```python
from build123d import *

# Parameters (mm, degrees)
ESQUISSE1_W                  = 40
ESQUISSE1_H                  = 50
BOSS_EXTRU_1_DEPTH           = 10
ENL_V_MAT_EXTRU_1_DEPTH      = 65.807406984
ENL_V_MAT_EXTRU_1_DEPTH_BACK = 65.807406984
ESQUISSE2_R                  = 3.4
ESQUISSE2_R_2                = 3.5
CONG_1_R                     = 5


with BuildPart() as part:
    # Esquisse1 → Boss.-Extru.1 (new body)
    with BuildSketch(Plane.XY):
        with Locations((20, 25)):
            Rectangle(ESQUISSE1_W, ESQUISSE1_H)
    extrude(amount=BOSS_EXTRU_1_DEPTH)

    # Esquisse2 → Enlèv. mat.-Extru.1 (cut, two sides: drawn at the far end of the back side and taken through both)
    with BuildSketch(Plane.XY.offset(10).offset(-ENL_V_MAT_EXTRU_1_DEPTH_BACK)):
        with Locations((20, 25)):
            Circle(ESQUISSE2_R)
        with Locations((20, 7.5)):
            Circle(ESQUISSE2_R_2)
        with Locations(Location((20, 42.5, 0), (0, 0, 180))):
            Circle(ESQUISSE2_R_2)
    extrude(amount=ENL_V_MAT_EXTRU_1_DEPTH + ENL_V_MAT_EXTRU_1_DEPTH_BACK, mode=Mode.SUBTRACT)

    # Congé1
    cong_1_edges = [part.edges().sort_by_distance(p)[0] for p in [
        (0, 50, 5),
        (40, 50, 5),
        (40, 0, 5),
        (0, 0, 5),
    ]]
    fillet(cong_1_edges, radius=CONG_1_R)


solid = part.part
```
Work out the finished part from the listing and answer in its coordinate system (mm). Give positions to 0.01 mm unless a question says otherwise; leave off trailing zeros. Loops run counter-clockwise (first coordinate to the right, second up) from the corner with the lowest first, then second, coordinate; pieces in that order, holes last. Notation, with made-up numbers: (-13, 12.5) -> (44, 12.5) arc R27 ccw to (44, 30.5) -> close; hole circle Ø11 at (-2, 30.25). An arc over 180 degrees is marked (long way). Put each result on its own line as item: value. Start each with the question number.
Item 1: The part is cut by section D-D (y = 25). Give the vertices of the cut face in (x, z).
Item 2: The part is cut by section C-C (z = 6.75). Give the vertices of the cut face in (x, y).
Item 3: Find the intervals of material crossed by L1, parallel to Y at x = 20, z = 5; L2, parallel to X at y = 7.5, z = 6.25; L3, parallel to X at y = 25, z = 8, in increasing order. Write a range as [from, to].
Item 4: The part is cut by section B-B (y = 7.5). Give the vertices of the cut face in (x, z).
Item 5: The part is cut by section A-A (x = 20). Give the vertices of the cut face in (y, z), then the cut area to 3 significant figures.
Answers below:
1. outline: (0, 0) -> (16.6, 0) -> (16.6, 10) -> (0, 10) -> close; (23.4, 0) -> (40, 0) -> (40, 10) -> (23.4, 10) -> close
2. outline: (0, 5) arc R5 ccw to (5, 0) -> (35, 0) arc R5 ccw to (40, 5) -> (40, 45) arc R5 ccw to (35, 50) -> (5, 50) arc R5 ccw to (0, 45) -> close; hole circle Ø7 at (20, 7.5); hole circle Ø7 at (20, 42.5); hole circle Ø6.8 at (20, 25)
3. L1: [0, 4], [11, 21.6], [28.4, 39], [46, 50]
3. L2: [0, 16.5], [23.5, 40]
3. L3: [0, 16.6], [23.4, 40]
4. outline: (0, 0) -> (16.5, 0) -> (16.5, 10) -> (0, 10) -> close; (23.5, 0) -> (40, 0) -> (40, 10) -> (23.5, 10) -> close
5. outline: (0, 0) -> (4, 0) -> (4, 10) -> (0, 10) -> close; (11, 0) -> (21.6, 0) -> (21.6, 10) -> (11, 10) -> close; (28.4, 0) -> (39, 0) -> (39, 10) -> (28.4, 10) -> close; (46, 0) -> (50, 0) -> (50, 10) -> (46, 10) -> close
5. area: 292 mm2
